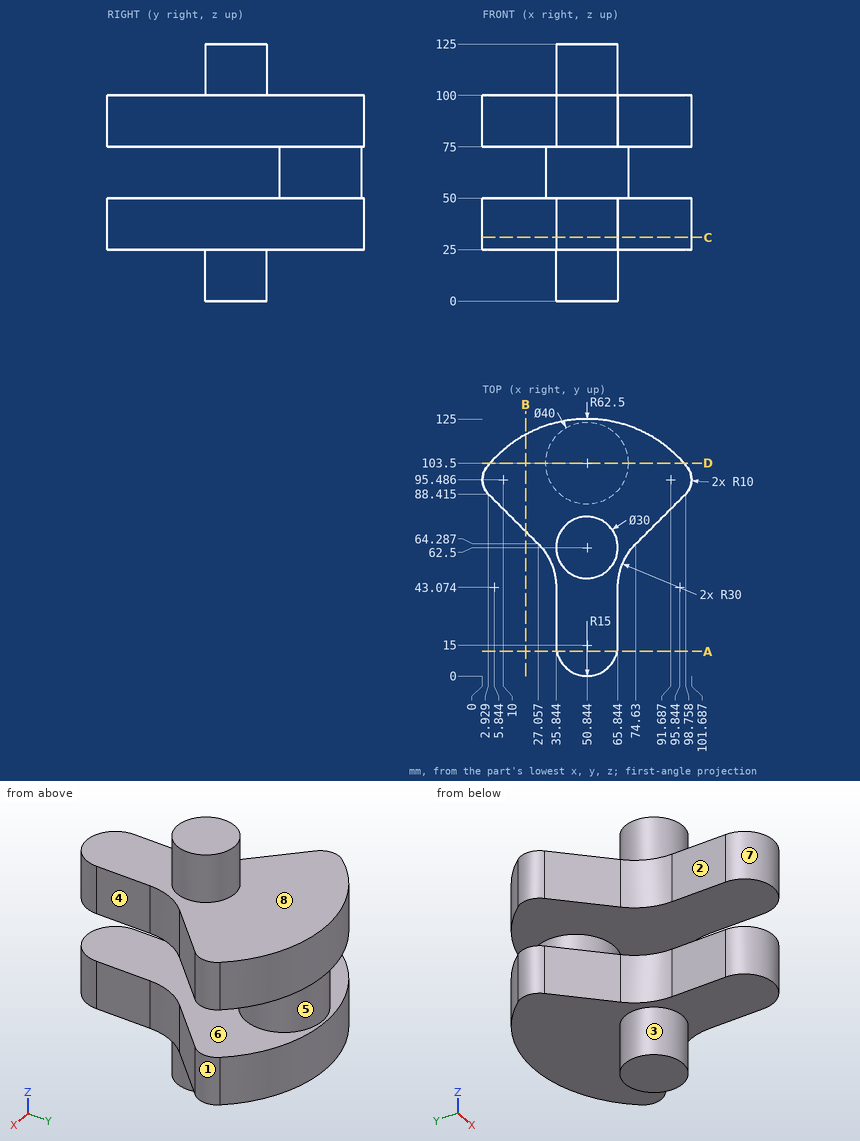
Check sheet for the drawn part. Datum: minimum x, y, z corner. Units: mm. A direction names the side the tool comes from. Round coordinates to 2 decimals unless told otherwise and drop trailing zeros. Write each loop counter-clockwise with the first axis right and the second up, starting at its lowest first coordinate (ties: lowest second). Pieces come first, ordered by that corner, then holes. Notation, with made-up numbers: (26, -6) -> (51, -6) arc R23 cw to (51, 33) -> close; hole circle Ø1 at (45, -26). An arc over 180 degrees is marked (long way). Write each question's results on one line, items separated by ' | '.
Q1. Sectioned sample at C-C, the plane z = 31. Record the boundary of the cut face in (x, y) (1 decimal).
Derived:
outline: (2.2, 101.8) arc R10 ccw to (2.9, 88.4) -> (27.1, 64.3) arc R30 cw to (35.8, 43.1) -> (35.8, 15) arc R15 ccw to (65.8, 15) -> (65.8, 43.1) arc R30 cw to (74.6, 64.3) -> (98.8, 88.4) arc R10 ccw to (99.5, 101.8) arc R62.5 ccw to start
Q2. Sectioned sample at D-D, the plane y = 103.5. Record the boundary of the cut face in (x, z).
Derived:
outline: (3.67, 25) -> (98.02, 25) -> (98.02, 50) -> (70.84, 50) -> (70.84, 75) -> (98.02, 75) -> (98.02, 100) -> (3.67, 100) -> (3.67, 75) -> (30.84, 75) -> (30.84, 50) -> (3.67, 50) -> close
Q3. Access from +Z, -Z, +X, -X, +Y, -Y to the whole of each face (thin tool, end or side, straight path). Record for the marked faces 1, 2, 3 and 4.
Derived:
face 1: +Z, -Z, +X | face 2: +Z, -Z, -X, -Y | face 3: -Z | face 4: +Z, -Z, +X, -Y
Q4. Draft check along Z on the marked faces 5, 6, 7 and 8. Enter one of: released by +Z, released by -Z, zero draft, split by the parting line, or undercut.
Derived:
face 5: undercut | face 6: undercut | face 7: zero draft | face 8: released by +Z
Q5. Thickness scan on probe 1 along Z at (x, y) = (32, 80); probe 2 along Z at (x, y) = (44.5, 63); probe 3 along Z at (x, y) = (38, 114). Record the ranges inside material, lowest first.
Derived:
probe 1: z = 25 to 50, 75 to 100 | probe 2: z = 0 to 50, 75 to 125 | probe 3: z = 25 to 100
Q6. Sectioned sample at B-B, the plane x = 21. Record the boundary of the cut face in (y, z) (1 decimal), and give its area (3 significant figures).
Derived:
outline: (70.3, 25) -> (117.4, 25) -> (117.4, 50) -> (70.3, 50) -> close; (70.3, 75) -> (117.4, 75) -> (117.4, 100) -> (70.3, 100) -> close | area: 2,350 mm²
Q7. Go/stop test with flat-tipped pins: pin 1 Ø12 at (x, z) = (44.5, 107) entering from +Y; pin 2 Ø1 at (x, z) = (87.5, 84) entering from +Y; pin 3 Ø3 at (y, z) = (44.5, 102) entering from +X; pin 4 Ø5 at (y, z) = (19, 39.5) entering from -X. Record where each tip stops, or that it passes through.
Derived:
pin 1: stops at y = 77.5 | pin 2: stops at y = 113.48 | pin 3: passes through | pin 4: stops at x = 35.84
Q8. Sectioned sample at A-A, the plane y = 12. Record the boundary of the cut face in (x, z), and give its area (3 significant figures).
Derived:
outline: (36.15, 25) -> (65.54, 25) -> (65.54, 50) -> (36.15, 50) -> close; (36.15, 75) -> (65.54, 75) -> (65.54, 100) -> (36.15, 100) -> close | area: 1,470 mm²
